from build123d import *

# Parameters (mm, degrees)
F0_W     = 83.9999988675
F0_H     = 63.9999988675
F0_W_2   = 36
F0_H_2   = 40
F1_DEPTH = 25
F2_W     = 73.9999988675
F2_H     = 53.9999988675
F3_DEPTH = 20
F4_R     = 6.2782984732
F5_DEPTH = 100


with BuildPart() as f1:
    # F0 (on Top) → F1 (new body)
    with BuildSketch(Plane.XY):
        with Locations((-12.5897452821, 0)):
            Rectangle(F0_W, F0_H)
        with Locations((-23.5897447158, 0)):
            Rectangle(F0_W_2, F0_H_2, mode=Mode.SUBTRACT)
    extrude(amount=F1_DEPTH)

    # F2 (on face) → F3 (cut)
    with BuildSketch(Plane.XY.offset(25)):
        with Locations((-12.5897452821, 0)):
            Rectangle(F2_W, F2_H)
    extrude(amount=-F3_DEPTH, mode=Mode.SUBTRACT)

    # F4 (on face) → F5 (cut)
    with BuildSketch(Plane(origin=(-54.5897447158, 0, 0), x_dir=(0, -1, 0), z_dir=(-1, 0, 0))):
        with Locations((0, 25)):
            Circle(F4_R)
    extrude(amount=-F5_DEPTH, mode=Mode.SUBTRACT)


solid = f1.part
Design review of the part built by this model. Coordinates are the model's own, in mm. A direction names the side the tool comes from. Round coordinates to 2 decimals unless told otherwise and drop trailing zeros. Order: outer loops, then holes, each group sorted by start corner. A loop starts at its lowest first (then second) coordinate and runs counter-clockwise, first axis right, second up. Notation, with made-up numbers: M 57.25,45 L 103.25,45 A16 ccw 103.25,53 Z; hole C 50,77 d1. An arc over 180 degrees is marked long. Answer as CSV lines item,"result". Start each with the question number.
1) Add section C-C (z = 3.5). Give the boundary of the cut face in (x, y), then the cut area to 3 significant figures.
2) Add section D-D (z = 22.5). Give the boundary of the cut face in (x, y), then the cut area to 3 significant figures.
3) Add section A-A (x = -9.5). Give the boundary of the cut face in (y, z).
4) Add section B-B (y = 0). Give the boundary of the cut face in (x, z), then the cut area to 3 significant figures.
5) For pin 1 Ø3 at (x, y) = (14, 23) entering from +Z, flat-tipped, find the tip position at first contact; note if it passes through.
6) Tool access review of faces 1 (the face through (-5, 0, 5)), 2 (the face through (-24, 20, 2)), 3 (the face through (-13, -29, 25)): name each direction out of +Z, -Z, +X, -X, +Y, -Y from which nothing blocks a thin tool from reaching the whole face with its end or side.
7) Wall thickness on line 1 along Y through (x, z) = (13.5, 23.25); line 2 along X through (y, z) = (-6.5, 23.5); line 3 along X through (y, z) = (12.5, 2): over which ranges is each line inside the solid? List them lowest first. Write a range as [from, to].
8) The part is to be moulded in two halves that separate along Y. For faces 4 (the face through (-13, -32, 12)), 5 (the face through (-5.59, 0, 2)), 6 (the face through (-54.59, 0, 12)), say which applies: +Y half, -Y half, draft (parallel to the pull), parting line (faces both ways), or undercut.
Resolved:
1,outline,"M -54.59,-32 L 29.41,-32 L 29.41,32 L -54.59,32 Z; hole M -41.59,-20 L -5.59,-20 L -5.59,20 L -41.59,20 Z"
1,area,"3,940 mm^2"
2,outline,"M -54.59,-32 L 29.41,-32 L 29.41,-5.76 L 24.41,-5.76 L 24.41,-27 L -49.59,-27 L -49.59,-5.76 L -54.59,-5.76 Z; M -54.59,5.76 L -49.59,5.76 L -49.59,27 L 24.41,27 L 24.41,5.76 L 29.41,5.76 L 29.41,32 L -54.59,32 Z"
2,area,"1,260 mm^2"
3,outline,"M -32,0 L -20,0 L -20,5 L -27,5 L -27,25 L -32,25 Z; M 20,0 L 32,0 L 32,25 L 27,25 L 27,5 L 20,5 Z"
4,outline,"M -54.59,0 L -41.59,0 L -41.59,5 L -49.59,5 L -49.59,18.72 L -54.59,18.72 Z; M -5.59,0 L 29.41,0 L 29.41,18.72 L 24.41,18.72 L 24.41,5 L -5.59,5 Z"
4,area,"377 mm^2"
5,pin 1,"z = 5"
6,face 1,"+Z"
6,face 2,"+Z, -Z"
6,face 3,"+Z, +X, -X, +Y, -Y"
7,line 1,"[-32, -27], [27, 32]"
7,line 2,"[-54.59, -49.59], [24.41, 29.41]"
7,line 3,"[-54.59, -41.59], [-5.59, 29.41]"
8,face 4,"-Y half"
8,face 5,"undercut"
8,face 6,"draft"
